Input: part model. Units: mm. Frame: model coordinates. A direction names the side the tool comes from. Coordinates: 2 decimals unless noted, no trailing zeros. Write each loop counter-clockwise with the first axis right and the second up, starting at its lowest first coordinate (ties: lowest second). Pieces come first, ordered by that corner, then holes. Notation, with made-up numbers: (4, 16) - (52, 16) arc R22 cw to (52, 47) - close; hole circle Ø10 at (41.25, 35.25). An arc over 180 degrees is marked (long way). Use CSV: the item, a comma, the result in double quotes.
```python
from build123d import *

# Parameters (mm, degrees)
SKETCH1_R           = 25.5
SKETCH1_R_2         = 22.5
SKETCH1_W           = 33.541019662
SKETCH1_H           = 30
BOSS_EXTRUDE1_DEPTH = 2.5
SKETCH2_W           = 1.5
SKETCH2_H           = 1.5
SKETCH2_W_2         = 41
BOSS_EXTRUDE2_DEPTH = 5
FILLET1_R           = 2.54
SKETCH3_W           = 10
SKETCH3_H           = 1.5
CUT_EXTRUDE1_DEPTH  = 5
SKETCH4_W           = 7
SKETCH4_H           = 3
BOSS_EXTRUDE3_DEPTH = 35
FILLET2_R           = 1.5
FILLET3_R           = 1.5
SKETCH5_W           = 11.5
SKETCH5_H           = 0.25
SKETCH5_H_2         = 1.25
SKETCH5_W_2         = 2
SKETCH5_H_3         = 7.25
BOSS_EXTRUDE5_DEPTH = 35
FILLET4_R           = 1.5
FILLET5_R           = 1.5
FILLET6_R           = 1
SKETCH6_W           = 9
SKETCH6_H           = 10
CUT_EXTRUDE3_DEPTH  = 19.76
FILLET7_R           = 1


with BuildPart() as part:
    # Sketch1 → Boss-Extrude1 (new body)
    # profile 1 of 4: a face of its own
    with BuildSketch(Plane(origin=(0, 0, 0), x_dir=(1, 0, 0), z_dir=(0, 1, 0))):
        with Locations(Location((0, 0, 0), (0, 0, 270))):
            Circle(SKETCH1_R)
        Circle(SKETCH1_R_2, mode=Mode.SUBTRACT)
    # profile 2 of 4: a face of its own
    with BuildSketch(Plane(origin=(0, 0, 0), x_dir=(1, 0, 0), z_dir=(0, 1, 0))):
        Rectangle(SKETCH1_W, SKETCH1_H)
    # profile 3 of 4: a face of its own
    with BuildSketch(Plane(origin=(0, 0, 0), x_dir=(1, 0, 0), z_dir=(0, 1, 0))):
        with BuildLine():
            ThreePointArc((22.5, 0), (21.018878077, 8.02849702), (16.770509831, 15))
            Line((16.770509831, 15), (16.770509831, -15))
            ThreePointArc((16.770509831, -15), (21.018878077, -8.02849702), (22.5, 0))
        make_face()
    # profile 4 of 4: a face of its own
    with BuildSketch(Plane(origin=(0, 0, 0), x_dir=(1, 0, 0), z_dir=(0, 1, 0))):
        with BuildLine():
            Line((-16.770509831, -15), (-16.770509831, 15))
            ThreePointArc((-16.770509831, 15), (-22.5, 0), (-16.770509831, -15))
        make_face()
    extrude(amount=BOSS_EXTRUDE1_DEPTH)

    # Sketch2 → Boss-Extrude2 (add)
    with BuildSketch(Plane(origin=(0, 2.5, 0), x_dir=(1, 0, 0), z_dir=(0, 1, 0))):
        Polygon((-20.5, -0.5), (-20.5, 5.5), (-20.5, 10.5), (-22, 10.5), (-22, -0.5), align=None)
        with Locations((-21.25, -1.25)):
            Rectangle(SKETCH2_W, SKETCH2_H)
        with Locations((0, -1.25)):
            Rectangle(SKETCH2_W_2, SKETCH2_H)
        Polygon((20.5, 10.5), (20.5, 5.5), (20.5, -0.5), (20.5, -2), (22, -2), (22, 12), (20.5, 12), align=None)
        Polygon((-20.5, 10.5), (20.5, 10.5), (20.5, 12), (-22, 12), (-22, 10.5), align=None)
    extrude(amount=BOSS_EXTRUDE2_DEPTH)

    # Fillet1
    fillet1_edges = [part.edges().sort_by_distance(p)[0] for p in [
        (-22, 5, -12),
        (-22, 5, 2),
        (22, 5, 2),
        (22, 5, -12),
    ]]
    fillet(fillet1_edges, radius=FILLET1_R)

    # Sketch3 → Cut-Extrude1 (cut)
    with BuildSketch(Plane(origin=(0, 7.5, 0), x_dir=(1, 0, 0), z_dir=(0, 1, 0))):
        with Locations((5.5, 11.25)):
            Rectangle(SKETCH3_W, SKETCH3_H)
    extrude(amount=-CUT_EXTRUDE1_DEPTH, mode=Mode.SUBTRACT)

    # Sketch4 → Boss-Extrude3 (add)
    with BuildSketch(Plane(origin=(0, 2.5, 0), x_dir=(1, 0, 0), z_dir=(0, 1, 0))):
        with Locations((-10, 13.5)):
            Rectangle(SKETCH4_W, SKETCH4_H)
    extrude(amount=BOSS_EXTRUDE3_DEPTH)

    # Fillet2
    fillet2_edges = [part.edges().sort_by_distance(p)[0] for p in [
        (-10, 7.5, -12),
        (-3, 2.5, -12),
        (-6.5, 2.5, -13.5),
        (-13.5, 2.5, -13.5),
        (0, 2.5, 2),
        (-22, 2.5, -5),
        (22, 2.5, -5),
        (-16.48, 2.5, -12),
        (-21.256051224, 2.5, 1.256051224),
        (21.256051224, 2.5, 1.256051224),
        (21.256051224, 2.5, -11.256051224),
        (-21.256051224, 2.5, -11.256051224),
        (14.98, 2.5, -12),
    ]]
    fillet(fillet2_edges, radius=FILLET2_R - 0.0001)  # a hair under: the kernel refuses the full size

    # Fillet3
    fillet3_edges = [part.edges().sort_by_distance(p)[0] for p in [
        (-10, 37.5, -12),
    ]]
    fillet(fillet3_edges, radius=FILLET3_R)

    # Sketch5 → Boss-Extrude5 (add)
    with BuildSketch(Plane(origin=(0, 2.5, 0), x_dir=(1, 0, 0), z_dir=(0, 1, 0))):
        with Locations((-5.75, -2.125)):
            Rectangle(SKETCH5_W, SKETCH5_H)
        with Locations((-5.75, -2.875)):
            Rectangle(SKETCH5_W, SKETCH5_H_2)
        with Locations((5.75, -2.875)):
            Rectangle(SKETCH5_W, SKETCH5_H_2)
        with Locations((5.75, -2.125)):
            Rectangle(SKETCH5_W, SKETCH5_H)
        Polygon((13.5, -2), (11.5, -2), (11.5, -2.25), (11.5, -3.5), (13.5, -3.5), align=None)
        with Locations((12.5, -7.125)):
            Rectangle(SKETCH5_W_2, SKETCH5_H_3)
        Polygon((11.5, -10.75), (-11.5, -10.75), (-13.5, -10.75), (-13.5, -12.825519341), (13.5, -12.825519341), (13.5, -10.75), align=None)
        with Locations((-12.5, -7.125)):
            Rectangle(SKETCH5_W_2, SKETCH5_H_3)
        Polygon((-11.5, -2.25), (-11.5, -2), (-13.5, -2), (-13.5, -3.5), (-11.5, -3.5), align=None)
    extrude(amount=BOSS_EXTRUDE5_DEPTH)

    # Fillet4
    fillet4_edges = [part.edges().sort_by_distance(p)[0] for p in [
        (0, 7.5, 2),
    ]]
    fillet(fillet4_edges, radius=FILLET4_R - 0.0001)  # a hair under: the kernel refuses the full size

    # Fillet5
    fillet5_edges = [part.edges().sort_by_distance(p)[0] for p in [
        (-13.5, 2.939310539, 2.439310539),
        (13.5, 2.939310539, 2.439310539),
        (13.5, 2.5, 8.16270967),
        (13.5, 5.74995, 2),
        (-13.5, 5.74995, 2),
        (0, 2.5, 12.825519341),
        (-13.5, 2.5, 8.16270967),
    ]]
    fillet(fillet5_edges, radius=FILLET5_R - 0.0001)  # a hair under: the kernel refuses the full size

    # Fillet6
    fillet6_edges = [part.edges().sort_by_distance(p)[0] for p in [
        (11.5, 20, 3.5),
        (11.5, 20, 10.75),
        (-11.5, 20, 10.75),
        (-11.5, 20, 3.5),
    ]]
    fillet(fillet6_edges, radius=FILLET6_R)

    # Sketch6 → Cut-Extrude3 (cut)
    with BuildSketch(Plane.XY.offset(12.825519341)):
        with Locations((-4.5, 25)):
            Rectangle(SKETCH6_W, SKETCH6_H)
        Polygon((9, 30), (0, 30), (0, 20), (-9, 20), (-9, 10), (9, 10), align=None)
    extrude(amount=-CUT_EXTRUDE3_DEPTH, mode=Mode.SUBTRACT)

    # Fillet7
    fillet7_edges = [part.edges().sort_by_distance(p)[0] for p in [
        (-9, 30, 11.78775967),
        (9, 30, 11.78775967),
        (9, 10, 11.78775967),
        (-9, 10, 11.78775967),
        (-9, 30, 2.75),
        (9, 30, 2.75),
        (9, 10, 2.75),
        (-9, 10, 2.75),
    ]]
    fillet(fillet7_edges, radius=FILLET7_R)


solid = part.part
```
(1) Draft query along X for faces 1 (the flat face through (-17, 6, 2)), 2 (the flat face through (9, 20, 12)), 3 (the cylindrical face through (-21.236, 5.774, 1.276)), 4 (the flat face through (10.5, 5, -11)). Return one class per face: pulls with the +X half, pulls with the -X half, needs draft (parallel to the pull), parting line crosses it, or undercut.
Check values:
face 1,"needs draft"
face 2,"undercut"
face 3,"pulls with the -X half"
face 4,"undercut"
(2) Cut plane A-A on y = 33.5. Return loops of the section in (x, z), and give its area (3 significant figures).
Check values:
outline,"(-13.5, -15) - (-6.5, -15) - (-6.5, -12) - (-13.5, -12) - close; (-13.5, 2) - (13.5, 2) - (13.5, 12.83) - (-13.5, 12.83) - close; hole (-11.5, 4.5) arc R1 ccw to (-10.5, 3.5) - (10.5, 3.5) arc R1 ccw to (11.5, 4.5) - (11.5, 9.75) arc R1 ccw to (10.5, 10.75) - (-10.5, 10.75) arc R1 ccw to (-11.5, 9.75) - close"
area,"147 mm^2"
(3) Ray query, probe 1 along Z at (x, y) = (-10.5, 29.5); probe 2 along Z at (x, y) = (-10, 5); probe 3 along Z at (x, y) = (5, 32). Return the intervals inside material, ascending. Write a range as from..to.
Check values:
probe 1,"-15..-12, 2..3.5, 10.75..12.83"
probe 2,"-15..-10.5, 0.5..3.5, 10.75..12.83"
probe 3,"2..3.5, 10.75..12.83"
(4) Pin query (flat end, axial travel): pin 1 Ø1.8 at (x, y) = (18, 6) entering from +Z; pin 2 Ø2.5 at (x, y) = (2.5, 6) entering from -Z; pin 3 Ø10 at (y, z) = (13, 8) entering from -X. Return the tip coordinate at first contact, or that it passes through.
Check values:
pin 1,"z = 2"
pin 2,"z = 0.5"
pin 3,"x = -13.5"
(5) Reachability of faces 5 (the cylindrical face through (13.93, 5.77, 2.45)), 6 (the cylindrical face through (-17.2, 2.93, 2.45)), 7 (the flat face through (0, 2.5, 7)) from +Z, -Z, +X, -X, +Y, -Y: full face, straight path, thin tool, end or side. Return the list, or none.
Check values:
face 5,"+Z, +X, +Y"
face 6,"+Z, -X, +Y"
face 7,"+Y"
(6) Cut plane C-C on z = 8. Return loops of the section in (x, y), and give its area (3 significant figures).
Check values:
outline,"(-24.21, 0) - (24.21, 0) - (24.21, 2.5) - (15, 2.5) arc R1.5 cw to (13.5, 4) - (13.5, 37.5) - (11.5, 37.5) - (11.5, 2.5) - (-11.5, 2.5) - (-11.5, 37.5) - (-13.5, 37.5) - (-13.5, 4) arc R1.5 cw to (-15, 2.5) - (-24.21, 2.5) - close"
area,"262 mm^2"
(7) Cut plane D-D on x = -1.5. State how many separate pieces and enclosed holes the cut face has, and give its area (3 significant figures).
Check values:
separate pieces,"5"
enclosed holes,"0"
area,"160 mm^2"
(8) Cut plane B-B on y = 20. Return loops of the section in (x, z).
Check values:
outline,"(-13.5, -15) - (-6.5, -15) - (-6.5, -12) - (-13.5, -12) - close; (-13.5, 2) - (-9, 2) - (-9, 3.5) - (-10.5, 3.5) arc R1 cw to (-11.5, 4.5) - (-11.5, 9.75) arc R1 cw to (-10.5, 10.75) - (-9, 10.75) - (-9, 12.83) - (-13.5, 12.83) - close; (9, 2) - (13.5, 2) - (13.5, 12.83) - (9, 12.83) - (9, 10.75) - (10.5, 10.75) arc R1 cw to (11.5, 9.75) - (11.5, 4.5) arc R1 cw to (10.5, 3.5) - (9, 3.5) - close"
